from build123d import *

# Parameters (mm, degrees)
SKETCH1_R           = 1
SKETCH1_W           = 0.508
SKETCH1_H           = 0.508
BOSS_EXTRUDE1_DEPTH = 12.5


with BuildPart() as part:
    # Sketch1 → Boss-Extrude1 (new, symmetric)
    with BuildSketch(Plane.XY):
        Circle(SKETCH1_R)
        with Locations((0, 1.221204218)):
            Rectangle(SKETCH1_W, SKETCH1_H)
        with Locations((0, -1.221204218)):
            Rectangle(SKETCH1_W, SKETCH1_H)
        with Locations((1.221204218, 0)):
            Rectangle(SKETCH1_W, SKETCH1_H)
        with Locations((-1.221204218, 0)):
            Rectangle(SKETCH1_W, SKETCH1_H)
    extrude(amount=BOSS_EXTRUDE1_DEPTH, both=True)


solid = part.part
Geometry check sheet. Reference: the model listing, model coordinates, mm. Give positions to 0.01 mm unless a question says otherwise; leave off trailing zeros. Loops run counter-clockwise (first coordinate to the right, second up) from the corner with the lowest first, then second, coordinate; pieces in that order, holes last. Notation, with made-up numbers: (75, 29.25) -> (105, 29.25) arc R22 cw to (105, 41.25) -> close; hole circle Ø11 at (-30, 5.25). An arc over 180 degrees is marked (long way). Answer in a Markdown table with one row per item. Add a question column.
1) Gauge pin test, flat end, axial feed: P1, Ø0.6, axis at x = 1, z = 3, coming from the -Y side. Record the tip position at first contact, or that the pin passes through.
2) Cross-section at B-B on y = 1.25. Record the boundary of the cut face in (x, z).
3) Cross-section at A-A on z = -5.25. Record the boundary of the cut face in (x, y).
4) Cross-section at C-C on x = -0.55. Record the boundary of the cut face in (y, z).
5) Material ranges on probe 1 along X at (y, z) = (1.3, 6.5); probe 2 along Y at (x, z) = (-0.5, -7.75), recorded low to high. Write a range as from..to.
Outcome:
| question | item | result |
|---|---|---|
| 1 | P1 | stops at y = -0.71 |
| 2 | outline | (-0.25, -12.5) -> (0.25, -12.5) -> (0.25, 12.5) -> (-0.25, 12.5) -> close |
| 3 | outline | (-1.48, -0.25) -> (-0.97, -0.25) arc R1 ccw to (-0.25, -0.97) -> (-0.25, -1.48) -> (0.25, -1.48) -> (0.25, -0.97) arc R1 ccw to (0.97, -0.25) -> (1.48, -0.25) -> (1.48, 0.25) -> (0.97, 0.25) arc R1 ccw to (0.25, 0.97) -> (0.25, 1.48) -> (-0.25, 1.48) -> (-0.25, 0.97) arc R1 ccw to (-0.97, 0.25) -> (-1.48, 0.25) -> close |
| 4 | outline | (-0.84, -12.5) -> (0.84, -12.5) -> (0.84, 12.5) -> (-0.84, 12.5) -> close |
| 5 | probe 1 | x = -0.25..0.25 |
| 5 | probe 2 | y = -0.87..0.87 |
